Study the drawing (mm; zero at the part's minimum x, y, z) and answer. A direction names the side the tool comes from. Coordinates: 2 decimals unless noted, no trailing zeros. Order: outer loops, then holes, each group sorted by start corner. A loop starts at its lowest first (then second) coordinate and runs counter-clockwise, first axis right, second up. Notation, with made-up numbers: (55.5, -24) - (65.5, -24) arc R11 ccw to (65.5, -19) - close; hole circle Ø8 at (23.5, -19). An arc over 180 degrees is marked (long way). Write item = value, one per line.
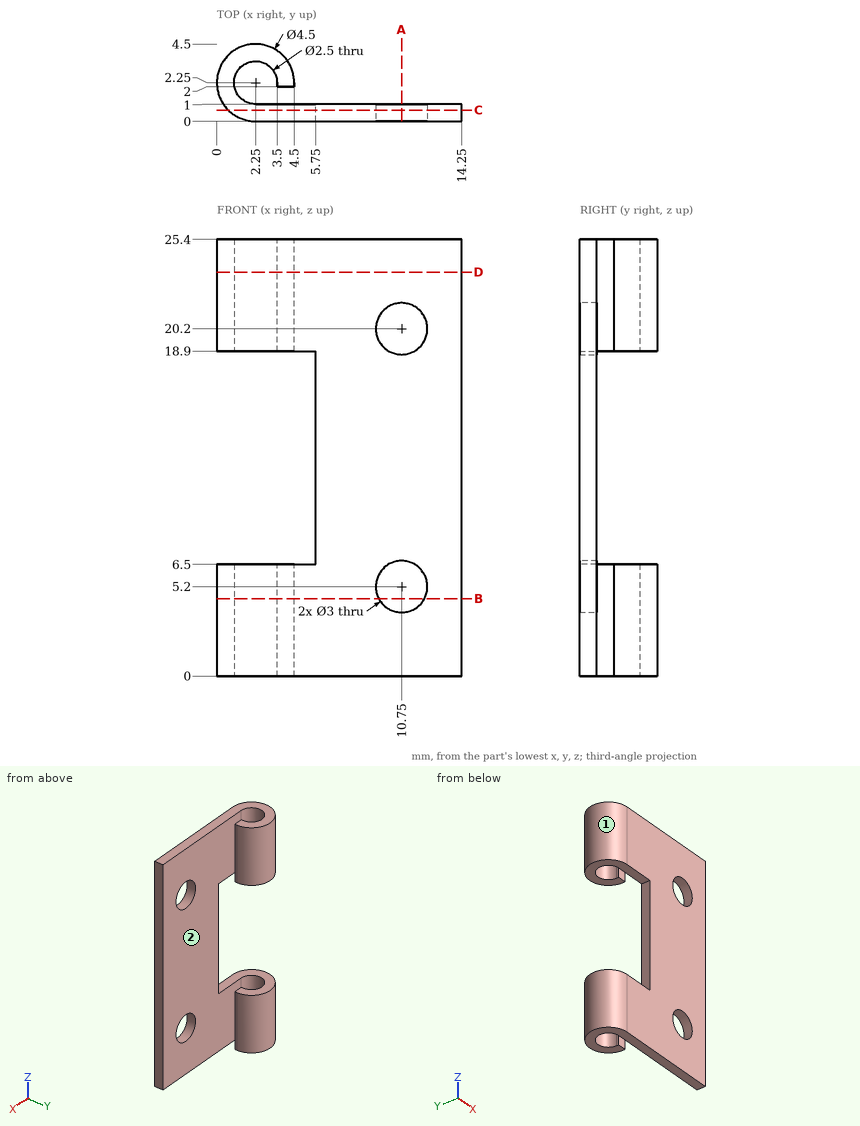
1) The part is cut by section A-A (x = 10.75). Determine the outline of the cut face in (y, z), and give its area (3 significant figures).
Returned:
outline = (0, 0) - (1, 0) - (1, 3.7) - (0, 3.7) - close; (0, 6.7) - (1, 6.7) - (1, 18.7) - (0, 18.7) - close; (0, 21.7) - (1, 21.7) - (1, 25.4) - (0, 25.4) - close
area = 19.4 mm^2
2) The part is cut by section D-D (z = 23.5). Determine the outline of the cut face in (x, y), and give its area (3 significant figures).
Returned:
outline = (2.25, 0) - (14.25, 0) - (14.25, 1) - (2.25, 1) arc R1.25 cw (long way) to (3.5, 2.25) - (3.5, 2) - (4.5, 2) - (4.5, 2.25) arc R2.25 ccw (long way) to start
area = 20.5 mm^2
3) The part is cut by section C-C (y = 0.65). Determine the outline of the cut face in (x, z).
Returned:
outline = (0.67, 0) - (14.25, 0) - (14.25, 25.4) - (0.67, 25.4) - (0.67, 18.9) - (5.75, 18.9) - (5.75, 6.5) - (0.67, 6.5) - close; hole circle Ø3 at (10.75, 5.2); hole circle Ø3 at (10.75, 20.2)
4) The part is cut by section B-B (z = 4.5). Determine the outline of the cut face in (x, y).
Returned:
outline = (2.25, 0) - (9.42, 0) - (9.42, 1) - (2.25, 1) arc R1.25 cw (long way) to (3.5, 2.25) - (3.5, 2) - (4.5, 2) - (4.5, 2.25) arc R2.25 ccw (long way) to start; (12.08, 0) - (14.25, 0) - (14.25, 1) - (12.08, 1) - close
5) For the marked faces 1 and 2, determine the directions among +Z, -Z, +X, -X, +Y, -Y from which every point of the face is accessible in a straight line to the end or side of a thin tool.
Returned:
face_1 = +Z, -Z
face_2 = +Z, -Z, +X
6) Flat-ended cylindrical pins translate along their axes: pin 1 Ø1.5 at (x, z) = (7.5, 4.5) entering from +Y; pin 2 Ø0.5 at (y, z) = (0.5, 14) entering from -X. Find the tip coordinate at first contact, or state that the pin passes through.
Returned:
pin_1 = 1
pin_2 = 5.75
7) Straight lines are drawn through the part: line 1 along X through (y, z) = (2.25, 1.5); line 2 along Y through (x, z) = (6, 3.5); line 3 along X through (y, z) = (2.85, 5.25). For each, find the intervals that lie inside material, in ascending order. Write a range as from..to.
Returned:
line_1 = 0..1, 3.5..4.5
line_2 = 0..1
line_3 = 0.08..1.15, 3.35..4.42
